from build123d import *

# Parameters (mm, degrees)
SKETCH1_W           = 80
SKETCH1_H           = 80.4
BOSS_EXTRUDE1_DEPTH = 4
SKETCH3_W           = 70
SKETCH3_H           = 40.2
BOSS_EXTRUDE3_DEPTH = 9
SKETCH4_R           = 1.375
CUT_EXTRUDE1_DEPTH  = 19
CUT_EXTRUDE4_REACH  = 60.181
SKETCH6_W           = 62
SKETCH6_H           = 35.2
SKETCH7_W           = 72
SKETCH7_H           = 80.4
SKETCH7_W_2         = 60
SKETCH7_H_2         = 68.4
BOSS_EXTRUDE4_DEPTH = 40
SKETCH9_R           = 1.2
CUT_EXTRUDE5_DEPTH  = 10
SKETCH10_W          = 70.4
SKETCH10_H          = 30
CUT_EXTRUDE6_DEPTH  = 10
CUT_EXTRUDE7_DEPTH  = 17
FILLET1_R           = 2.4


with BuildPart() as part:
    # Sketch1 → Boss-Extrude1 (new body)
    with BuildSketch(Plane(origin=(0, 0, 0), x_dir=(1, 0, 0), z_dir=(0, 1, 0))):
        Rectangle(SKETCH1_W, SKETCH1_H)
    extrude(amount=BOSS_EXTRUDE1_DEPTH)

    # Sketch3 → Boss-Extrude3 (add)
    with BuildSketch(Plane.XZ):
        with Locations((5, -20.1)):
            Rectangle(SKETCH3_W, SKETCH3_H)
    extrude(amount=BOSS_EXTRUDE3_DEPTH)

    # Sketch4 → Cut-Extrude1 (cut)
    with BuildSketch(Plane.XZ.offset(9)):
        with Locations(Location((-36.5, 24, 0), (0, 0, 270))):
            Circle(SKETCH4_R)
        with Locations(Location((-36.5, -24, 0), (0, 0, 270))):
            Circle(SKETCH4_R)
    extrude(amount=-CUT_EXTRUDE1_DEPTH, mode=Mode.SUBTRACT)

    # Sketch6 → Cut-Extrude4 (cut, up to next)
    with BuildSketch(Plane(origin=(0, 4, 0), x_dir=(1, 0, 0), z_dir=(0, 1, 0)), mode=Mode.PRIVATE) as cut_extrude4_sk1:
        with Locations((4, -17.6)):
            Rectangle(SKETCH6_W, SKETCH6_H)
    cut_extrude4_tool1 = extrude(cut_extrude4_sk1.sketch, amount=-CUT_EXTRUDE4_REACH, mode=Mode.PRIVATE) & part.part
    add(cut_extrude4_tool1.solids().sort_by_distance((4, 4, 17.6))[0], mode=Mode.SUBTRACT)

    # Sketch7 → Boss-Extrude4 (add)
    with BuildSketch(Plane.XZ.offset(-4)):
        with Locations((4, 0)):
            Rectangle(SKETCH7_W, SKETCH7_H)
        with Locations((4, 0)):
            Rectangle(SKETCH7_W_2, SKETCH7_H_2, mode=Mode.SUBTRACT)
    extrude(amount=-BOSS_EXTRUDE4_DEPTH)

    # Sketch9 → Cut-Extrude5 (cut)
    with BuildSketch(Plane(origin=(0, 44, 0), x_dir=(1, 0, 0), z_dir=(0, 1, 0))):
        with Locations(Location((-29, 37.2, 0), (0, 0, 270))):
            Circle(SKETCH9_R)
        with Locations(Location((37, 37.2, 0), (0, 0, 270))):
            Circle(SKETCH9_R)
        with Locations(Location((37, -37.2, 0), (0, 0, 270))):
            Circle(SKETCH9_R)
        with Locations(Location((-29, -37.2, 0), (0, 0, 270))):
            Circle(SKETCH9_R)
    extrude(amount=-CUT_EXTRUDE5_DEPTH, mode=Mode.SUBTRACT)

    # Sketch10 → Cut-Extrude6 (cut)
    with BuildSketch(Plane.ZY.offset(32)):
        with Locations((0, 24)):
            Rectangle(SKETCH10_W, SKETCH10_H)
    extrude(amount=-CUT_EXTRUDE6_DEPTH, mode=Mode.SUBTRACT)

    # Sketch11 → Cut-Extrude7 (cut)
    with BuildSketch(Plane(origin=(0, 9, 0), x_dir=(1, 0, 0), z_dir=(0, 1, 0))):
        Polygon((-32, 0), (-32, -35.2), (-23.981492028, -35.2), (-23.981492028, -34.2), (-26, -34.2), (-26, 0), align=None)
    extrude(amount=-CUT_EXTRUDE7_DEPTH, mode=Mode.SUBTRACT)

    # Fillet1
    # the kernel refuses this fillet: 2.4 mm, written as the material it adds along each edge
    with BuildSketch(Plane(origin=(-32, 4, 0), x_dir=(0, 1, 0), z_dir=(0, 0, -1)), Plane(origin=(-30, 0, 0), x_dir=(-1, 0, 0), z_dir=(0, 0, -1))) as fillet1_piece_1:
        with BuildLine():
            CenterArc((FILLET1_R, -FILLET1_R), FILLET1_R, 90, 90)
            Line((0, -FILLET1_R), (0, 0))
            Line((0, 0), (FILLET1_R, 0))
        make_face()
    extrude(amount=40.2)


solid = part.part
The model under review builds one solid part; all positions refer to its coordinate system, in mm. A direction names the side the tool comes from. Round coordinates to 2 decimals unless told otherwise and drop trailing zeros. Loops run counter-clockwise (first coordinate to the right, second up) from the corner with the lowest first, then second, coordinate; pieces in that order, holes last. Notation, with made-up numbers: (-39, 12) -> (-25, 12) arc R13 ccw to (-25, 23) -> close; hole circle Ø10 at (62, 43). An arc over 180 degrees is marked (long way). One line per question, with ' | ' between items. Start each with the question number.
Item 1: Draft analysis for pull direction X (two halves, no side actions). For faces 5 (the face through (5, -9, -20)), 6 (the face through (-32, 2, 17)), 7 (the face through (-32.684, 4.722, -19.819)), state which applies: +X half, -X half, draft (parallel to the pull), parting line (faces both ways), or undercut.
Item 2: Add section C-C, the plane x = -5. Write out the cut boundary in (y, z), then the cut area to 3 significant figures.
Item 3: Machinability: for faces 1 (the face through (-29, 39, 0)), 2 (the face through (-30, -6, -20)), 3 (the face through (4, 24, -34.2)), 4 (the face through (5, 4, 35)), which of the approach directions +Z, -Z, +X, -X, +Y, -Y give a long, thin tool a straight path to every point of the face, cutting with its end or side? Answer none if there is none.
Item 4: Add section B-B, the plane z = 30. Write out the cut boundary in (x, y), then the cut area to 3 significant figures.
Item 5: Add section D-D, the plane z = -12.5. Write out the cut boundary in (x, y), then the cut area to 3 significant figures.
Item 6: Add section A-A, the plane x = -36.5. Write out the cut boundary in (y, z) (3 decimals), then the cut area to 3 significant figures.
Item 7: For pin 1 (2.5 mm diameter, centred on x = -37, z = -16.5, fed in from +Y); pin 2 (8 mm diameter, centred on y = 15.5, z = -12, fed in from -X); pin 3 (0.5 mm diameter, centred on y = 26.5, z = 34.5, fed in from -X), all flat-tipped, find the tip position at first contact; note any pin that passes through.
Item 8: Wall thickness on line 1 along X through (y, z) = (1.65, 24) (3 decimals); line 2 along X through (y, z) = (40, -37.2); line 3 along Z through (x, y) = (-21, 2.5): over which ranges is each line inside the solid? List them lowest first. Write a range as [from, to].
Return value:
1) face 5: draft | face 6: undercut | face 7: -X half
2) outline: (-9, -40.2) -> (44, -40.2) -> (44, -34.2) -> (4, -34.2) -> (4, 0) -> (-9, 0) -> close; (0, 35.2) -> (4, 35.2) -> (4, 34.2) -> (44, 34.2) -> (44, 40.2) -> (0, 40.2) -> close | area: 1,020 mm2
3) face 1: -X | face 2: +Z, -Z, -X, -Y | face 3: +Y | face 4: -Y
4) outline: (-40, 0) -> (-32, 0) -> (-32, 4) -> (-40, 4) -> close; (-32, 39) -> (-26, 39) -> (-26, 44) -> (-32, 44) -> close; (34, 4) -> (35, 4) -> (35, 0) -> (40, 0) -> (40, 44) -> (34, 44) -> close | area: 322 mm2
5) outline: (-40, 0) -> (-32.4, 0) arc R2.4 cw to (-30, -2.4) -> (-30, -9) -> (40, -9) -> (40, 44) -> (34, 44) -> (34, 4) -> (-26, 4) -> (-26, 9) -> (-32, 9) -> (-32, 6.4) arc R2.4 cw to (-34.4, 4) -> (-40, 4) -> close; (-32, 39) -> (-26, 39) -> (-26, 44) -> (-32, 44) -> close | area: 1,250 mm2
6) outline: (0, -40.2) -> (4, -40.2) -> (4, -25.375) -> (0, -25.375) -> close; (0, -22.625) -> (4, -22.625) -> (4, 22.625) -> (0, 22.625) -> close; (0, 25.375) -> (4, 25.375) -> (4, 40.2) -> (0, 40.2) -> close | area: 300 mm2
7) pin 1: stops at y = 4 | pin 2: stops at x = 34 | pin 3: stops at x = -22
8) line 1: x = [-40, -37.875], [-35.125, -32], [35, 40] | line 2: x = [-32, -30.2], [-27.8, 35.8], [38.2, 40] | line 3: z = [-40.2, 0], [35.2, 40.2]
